from build123d import *

# Parameters (mm, degrees)
SKETCH_1_R      = 30
EXTRUDE_1_DEPTH = 7
SKETCH_2_R      = 15
EXTRUDE_2_DEPTH = 50
SKETCH_3_W      = 50
SKETCH_3_H      = 50
EXTRUDE_3_DEPTH = 30


with BuildPart() as part:
    # 스케치1 → 보스-돌출1 (new body)
    with BuildSketch(Plane.XY):
        Circle(SKETCH_1_R)
    extrude(amount=EXTRUDE_1_DEPTH)

    # 스케치2 → 보스-돌출2 (add)
    with BuildSketch(Plane.XY.offset(7)):
        Circle(SKETCH_2_R)
    extrude(amount=EXTRUDE_2_DEPTH)

    # 스케치3 → 보스-돌출3 (add)
    with BuildSketch(Plane.XY.offset(57)):
        Rectangle(SKETCH_3_W, SKETCH_3_H)
    extrude(amount=EXTRUDE_3_DEPTH)


solid = part.part
CAD build for the part. Positions are in the model's coordinates, mm. A direction names the side the tool comes from. Coordinates: 2 decimals unless noted, no trailing zeros. Order: outer loops, then holes, each group sorted by start corner. A loop starts at its lowest first (then second) coordinate and runs counter-clockwise, first axis right, second up. Notation, with made-up numbers: (-36.75, 59.25) -> (-27.75, 59.25) arc R6 cw to (-27.75, 70.25) -> close; hole circle Ø2 at (84.5, 45.5). An arc over 180 degrees is marked (long way). Answer in a Markdown table with one row per item.
1) Which spindle directions (+Z, -Z, +X, -X, +Y, -Y) get a long thin tool onto all of the face, cutting with end or side? Do faces 5 (the face through (25, 0, 72)), 6 (the face through (-11, 11, 57)), 7 (the face through (-25, 0, 72)). Say none if no direction does.
Check values:
| item | result |
|---|---|
| face 5 | +Z, +X, +Y, -Y |
| face 6 | none |
| face 7 | +Z, -X, +Y, -Y |
2) Mould opens along Z. For faces 1 (the face through (0, 0, 87)), 2 (the face through (0, 25, 72)), 3 (the face through (-14.985, 0.66, 31.65)), 4 (the face through (0, 0, 0)) say: pulls with the +Z half, pulls with the -Z half, needs draft (parallel to the pull), parting line crosses it, or undercut.
Check values:
| item | result |
|---|---|
| face 1 | pulls with the +Z half |
| face 2 | needs draft |
| face 3 | undercut |
| face 4 | pulls with the -Z half |
3) Band-saw the part on A-A (y = -24). List the corners of the cut face in (x, z), and give its area (3 significant figures).
Check values:
| item | result |
|---|---|
| outline | (-25, 57) -> (25, 57) -> (25, 87) -> (-25, 87) -> close; (-18, 0) -> (18, 0) -> (18, 7) -> (-18, 7) -> close |
| area | 1,750 mm2 |
4) Drill centre lines: line 1 (Z direction, x = 4.5, y = 22); line 2 (Y direction, x = 14, z = 66). Where is each one in solid material? Low to high.
Check values:
| item | result |
|---|---|
| line 1 | 0 to 7, 57 to 87 |
| line 2 | -25 to 25 |
5) Band-saw the part on B-B (x = 18.5). List the corners of the cut face in (y, z), and give its area (3 significant figures).
Check values:
| item | result |
|---|---|
| outline | (-25, 57) -> (25, 57) -> (25, 87) -> (-25, 87) -> close; (-23.62, 0) -> (23.62, 0) -> (23.62, 7) -> (-23.62, 7) -> close |
| area | 1,830 mm2 |
6) Band-saw the part on C-C (y = 0). List the corners of the cut face in (x, z).
Check values:
| item | result |
|---|---|
| outline | (-30, 0) -> (30, 0) -> (30, 7) -> (15, 7) -> (15, 57) -> (25, 57) -> (25, 87) -> (-25, 87) -> (-25, 57) -> (-15, 57) -> (-15, 7) -> (-30, 7) -> close |
7) Flat gauge pins, fed straight in: P1, Ø15, axis at y = -12, z = 78.5, coming from the -X side; P2, Ø24, axis at x = 3.5, z = 72.5, coming from the -Y side; P3, Ø8, axis at x = -11, z = 13, coming from the +Y side. Where does each tip first touch, or does it go through?
Check values:
| item | result |
|---|---|
| P1 | x = -25 |
| P2 | y = -25 |
| P3 | y = 13.27 |
